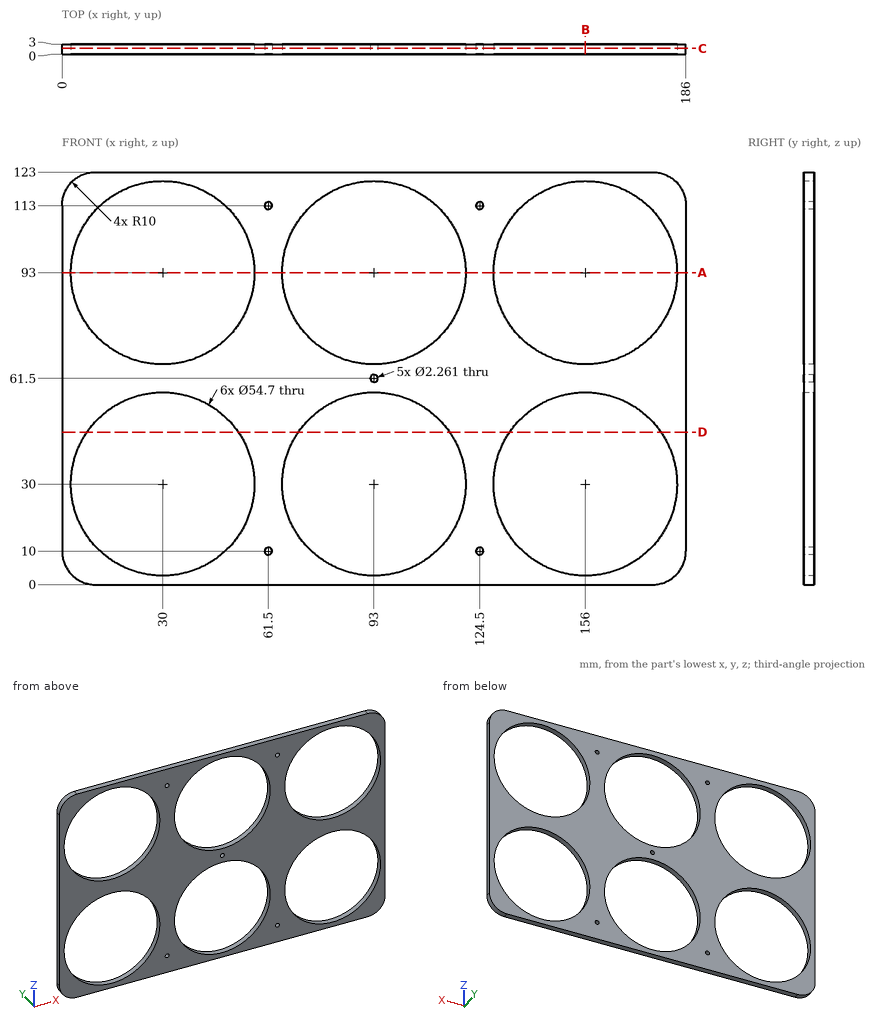
The figure shows three views and two pictorial views of one solid part (mm, origin at its lowest corner). Answer the questions. Coordinates: 2 decimals unless noted, no trailing zeros. Loops run counter-clockwise (first coordinate to the right, second up) from the corner with the lowest first, then second, coordinate; pieces in that order, holes last. Notation, with made-up numbers: (29.25, 34) -> (60.25, 34) arc R36 ccw to (60.25, 72) -> close; hole circle Ø2 at (12, 36.25). An arc over 180 degrees is marked (long way). Use one line per item in the form item = value. Start each with the question number.
Item 1: The part is cut by section B-B on x = 156. Determine the outline of the cut face in (y, z), then the cut area to 3 significant figures.
Item 2: The part is cut by section A-A on z = 93. Determine the outline of the cut face in (x, y).
Item 3: The part is cut by section C-C on y = 1.7. Count the separate pieces of the cut face and the enclosed holes in it, then the cut area to 3 significant figures.
Item 4: The part is cut by section D-D on z = 45.5. Determine the outline of the cut face in (x, y), then the cut area to 3 significant figures.
Item 5: Consider L1, parallel to X at y = 1.7, z = 30; L2, parallel to Z at x = 61.5, y = 1.9; L3, parallel to X at y = 0.8, z = 113 (1 decimal). Determine where each line is inside the solid, lowest interval first. Write a range as [from, to].
Answer key:
q1.outline = (0, 0) -> (3, 0) -> (3, 2.65) -> (0, 2.65) -> close; (0, 57.35) -> (3, 57.35) -> (3, 65.65) -> (0, 65.65) -> close; (0, 120.35) -> (3, 120.35) -> (3, 123) -> (0, 123) -> close
q1.area = 40.8 mm2
q2.outline = (0, 0) -> (2.65, 0) -> (2.65, 3) -> (0, 3) -> close; (57.35, 0) -> (65.65, 0) -> (65.65, 3) -> (57.35, 3) -> close; (120.35, 0) -> (128.65, 0) -> (128.65, 3) -> (120.35, 3) -> close; (183.35, 0) -> (186, 0) -> (186, 3) -> (183.35, 3) -> close
q3.separate_pieces = 1
q3.enclosed_holes = 11
q3.area = 8,670 mm2
q4.outline = (0, 0) -> (7.47, 0) -> (7.47, 3) -> (0, 3) -> close; (52.53, 0) -> (70.47, 0) -> (70.47, 3) -> (52.53, 3) -> close; (115.53, 0) -> (133.47, 0) -> (133.47, 3) -> (115.53, 3) -> close; (178.53, 0) -> (186, 0) -> (186, 3) -> (178.53, 3) -> close
q4.area = 152 mm2
q5.L1 = [0, 2.65], [57.35, 65.65], [120.35, 128.65], [183.35, 186]
q5.L2 = [0, 8.87], [11.13, 111.87], [114.13, 123]
q5.L3 = [0, 11.3], [48.7, 60.4], [62.6, 74.3], [111.7, 123.4], [125.6, 137.3], [174.7, 186]
